Geometry: final body of the model. Coordinates: model frame, mm. A direction names the side the tool comes from. Round coordinates to 2 decimals unless told otherwise and drop trailing zeros. Order: outer loops, then holes, each group sorted by start corner. A loop starts at its lowest first (then second) coordinate and runs counter-clockwise, first axis right, second up. Notation, with made-up numbers: (18.25, 8.5) -> (41.25, 8.5) arc R15 ccw to (41.25, 28.5) -> close; hole circle Ø2 at (20, -3.75). An arc over 180 degrees is marked (long way). Put each result on its own line as item: value.
Autodesk Inventor part; units mm, degrees
ref_plane "YZ Plane" through (0, 0, 0) normal (1, 0, 0) x (0, 1, 0)
ref_plane "XZ Plane" through (0, 0, 0) normal (0, 1, 0) x (-1, 0, 0)
ref_plane "XY Plane" through (0, 0, 0) normal (0, 0, 1) x (1, 0, 0)
sketch "Szkic1" plane through (0, 0, 0) normal (1, 0, 0) x (0, 1, 0)
  line L0 (5, 0) -> (-5, 0)
  line L1 (-5, 0) -> (-5, -19.25)
  line L2 (-5, -60) -> (5, -60)
  line L3 (5, -60) -> (5, 0)
  line L4 (5, 0) -> (5, -32)
  line L5 (5, 0) -> (5, -28.5)
  line L6 (-5, 0) -> (-5, -6)
  line L7 (-7.3, 0) -> (7.05, 0)
  line L8 (-5, 0) -> (-5, -33.2566)
  line L9 (-5, 0) -> (-5.25, 0)
  arc A0 (-5, -42.7434) -> (-5, -33.2566) centre (-5.25, -38) ccw
  line L10 (-5, -42.7434) -> (-5, -60)
  line L11 (-5, -28.75) -> (-5, -33.2566)
  line L12 (-5, -42.7434) -> (-5, -60)
  point P0 (0, 0)
  point P1 (0, 0)
  dimension "d0" = 10
  dimension "d1" = 60
  dimension "d44" = 38
  dimension "d48" = 4.75
revolve "Obrót2" add sketch "Szkic1" angle 360 about axis through (0, 5, 0) along (0, -1, 0)
sketch "Szkic4" plane through (0, 5, 0) normal (0, 1, 0) x (1, 0, 0)
  line L0 (0, 0) -> (0, 48)
  circle A0 centre (0, 48) radius 3.5
  circle A1 centre (-41.5692, 24) radius 3.5
  circle A2 centre (-41.5692, -24) radius 3.5
  circle A3 centre (0, -48) radius 3.5
  circle A4 centre (41.5692, -24) radius 3.5
  circle A5 centre (41.5692, 24) radius 3.5
  circle A6 centre (0, 0) radius 3
  dimension "d32" = 48
  dimension "d33" = 7
  dimension "d36" = 360
  dimension "d38" = 6
extrude "Wyciągnięcie proste5" cut sketch "Szkic4" against normal blind 5 contours A0 | A1 | A2 | A3 | A4 | A5
sketch "Szkic5" plane through (0, 5, 0) normal (0, 1, 0) x (1, 0, 0)
  circle A0 centre (0, 0) radius 3
  dimension "d41" = 6
extrude "Wyciągnięcie proste6" cut sketch "Szkic5" against normal blind 10
chamfer "Faza2" distance 0.5 angle 45 2 edges at (0, -5, 42.7434) (0, -5, 33.2566)
properties part number "Base"
1. Cut plane A-A on y = 3.5. Return loops of the section in (x, z), and give its area (3 significant figures).
Ans:
outline: circle Ø120 at (0, 0); hole circle Ø7 at (-41.57, -24); hole circle Ø7 at (-41.57, 24); hole circle Ø7 at (0, -48); hole circle Ø7 at (0, 48); hole circle Ø6 at (0, 0); hole circle Ø7 at (41.57, -24); hole circle Ø7 at (41.57, 24)
area: 11,100 mm²
2. Material intervals for probe 1 along Z at (x, y) = (-42, 4); probe 2 along X at (y, z) = (0.75, 24); probe 3 along Z at (x, y) = (-9, -1.25), sorted ascending.
Ans:
probe 1: -42.85 to -27.47, -20.53 to 20.53, 27.47 to 42.85
probe 2: -54.99 to -45.07, -38.07 to 38.07, 45.07 to 54.99
probe 3: -59.32 to -39.55, -34.28 to 34.28, 39.55 to 59.32
3. Set-up query: faces 1 (the face through (-3, 0, 0)), 2 (the face through (42, 0, 24)). Return all of +Z, -Z, +X, -X, +Y, -Y with unobstructed straight access to the full face (end or side cutting, diameter ignored); none if empty.
Ans:
face 1: +Y, -Y
face 2: +Y
4. Cut plane D-D on x = 47.5. Return loops of the section in (y, z), and give its area (3 significant figures).
Ans:
outline: (-5, -36.66) -> (5, -36.66) -> (5, 36.66) -> (-5, 36.66) -> close
area: 733 mm²
5. Cut plane C-C on y = -2.5. Return loops of the section in (x, z), and give its area (3 significant figures).
Ans:
outline: circle Ø120 at (0, 0); circle Ø68.25 at (0, 0); hole circle Ø83.75 at (0, 0); hole circle Ø6 at (0, 0)
area: 9,430 mm²
6. Draft query along X for faces 3 (the face through (-40, -5, -17)), 4 (the face through (-0.46, 2.54, 44.53)), 5 (the face through (-2.64, 0.07, 59.94)), 6 (the face through (0, 0, -48)). Return one class per face: +X half, -X half, draft (parallel to the pull), parting line (faces both ways), or undercut.
Ans:
face 3: draft
face 4: undercut
face 5: parting line
face 6: undercut
7. Cut plane B-B on z = 50. Return loops of the section in (x, y), and give its area (3 significant figures).
Ans:
outline: (-33.17, -5) -> (33.17, -5) -> (33.17, 5) -> (2.87, 5) -> (2.87, 0) -> (-2.87, 0) -> (-2.87, 5) -> (-33.17, 5) -> close
area: 635 mm²
8. Contact query for flat-ended pins moving along their axis: P1, Ø4, axis at x = 44.5, y = 1.5, coming from the +Z side; P2, Ø3.5, axis at x = -41, z = 24.5, coming from the +Y side; P3, Ø1.5, axis at x = -27.5, y = -2, coming from the -Z side; P4, Ø5, axis at x = 0, z = 0, coming from the +Y side. Output: stop coordinate, or through.
Ans:
P1: z = 42.35
P2: y = 0
P3: z = -53.71
P4: through
